Part model, mm, in its own coordinate system. Face numbers are marked on the shaded views. Give positions to 0.01 mm unless a question says otherwise; leave off trailing zeros.
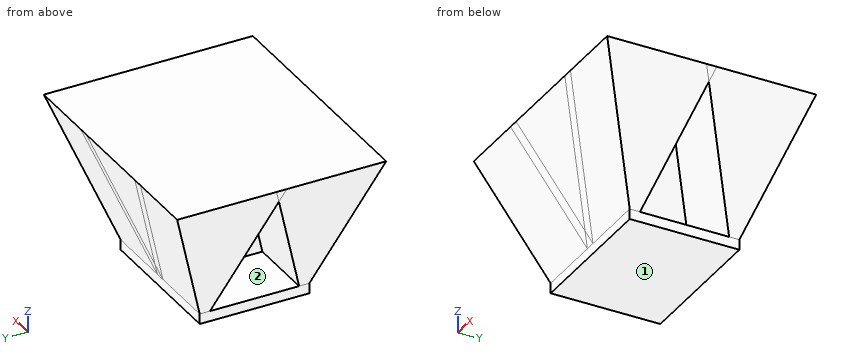
from build123d import *
from build123d.topology import SkipClean

# Parameters (mm, degrees)
SKETCH1_W           = 42.4
SKETCH1_H           = 32.12
BOSS_EXTRUDE1_DEPTH = 3
SKETCH2_W           = 42.4
SKETCH2_H           = 3
SKETCH2_W_2         = 3
SKETCH2_H_2         = 32.12
BOSS_EXTRUDE2_DEPTH = 40
BOSS_EXTRUDE2_TAPER = -20


with BuildPart() as part:
    # Sketch1 → Boss-Extrude1 (new body)
    with BuildSketch(Plane.XY):
        Rectangle(SKETCH1_W, SKETCH1_H)
    extrude(amount=BOSS_EXTRUDE1_DEPTH)

    # Sketch2 → Boss-Extrude2 (add)
    with SkipClean():  # the faces are left unmerged after this step: merging them gives an invalid solid
        with BuildSketch(Plane.XY.offset(3)):
            with Locations((0, 14.56)):
                Rectangle(SKETCH2_W, SKETCH2_H)
            with Locations((0, -14.56)):
                Rectangle(SKETCH2_W, SKETCH2_H)
            Rectangle(SKETCH2_W_2, SKETCH2_H_2)
        extrude(amount=BOSS_EXTRUDE2_DEPTH, taper=BOSS_EXTRUDE2_TAPER)
    add(part.part.scale(1), mode=Mode.REPLACE)  # the faces are merged on a copy


solid = part.part
1) Flat gauge pins, fed straight in: P1, Ø1.5, axis at x = 18.5, z = 15, coming from the +Y side; P2, Ø4, axis at x = 14.5, z = 38.5, coming from the +Y side; P3, Ø2, axis at x = 19.5, z = 8.5, coming from the +Y side. Where does each tip first touch, or does it go through?
Check result:
P1: stops at y = 20.7
P2: stops at y = 29.71
P3: stops at y = 18.43
2) Drill centre lines: L1, parallel to Y at x = 19.5, z = 15.5; L2, parallel to Y at x = 16.5, z = 22.5; L3, parallel to X at y = -8, z = 16. Where is each one in solid material? Low to high.
Check result:
L1: y = -20.61 to -8.51, 8.51 to 20.61
L2: y = -23.16 to -5.96, 5.96 to 23.16
L3: x = -6.23 to 6.23
3) Mould opens along Y. For the marked faces 1 and 2 say: +Y half, -Y half, draft (parallel to the pull), parting line (faces both ways), or undercut.
Check result:
face 1: draft
face 2: undercut
